Can you work these out from the drawing? Everything is in mm from the part's minimum corner. A direction names the side the tool comes from. Round coordinates to 2 decimals unless told otherwise and drop trailing zeros. Order: outer loops, then holes, each group sorted by start corner. A loop starts at its lowest first (then second) coordinate and runs counter-clockwise, first axis right, second up. Notation, with made-up numbers: (56, 23.5) - (92, 23.5) arc R22 cw to (92, 50.5) - close; hole circle Ø3 at (55.5, -4). An arc over 180 degrees is marked (long way). Answer as a JSON object with one key per item and string values.
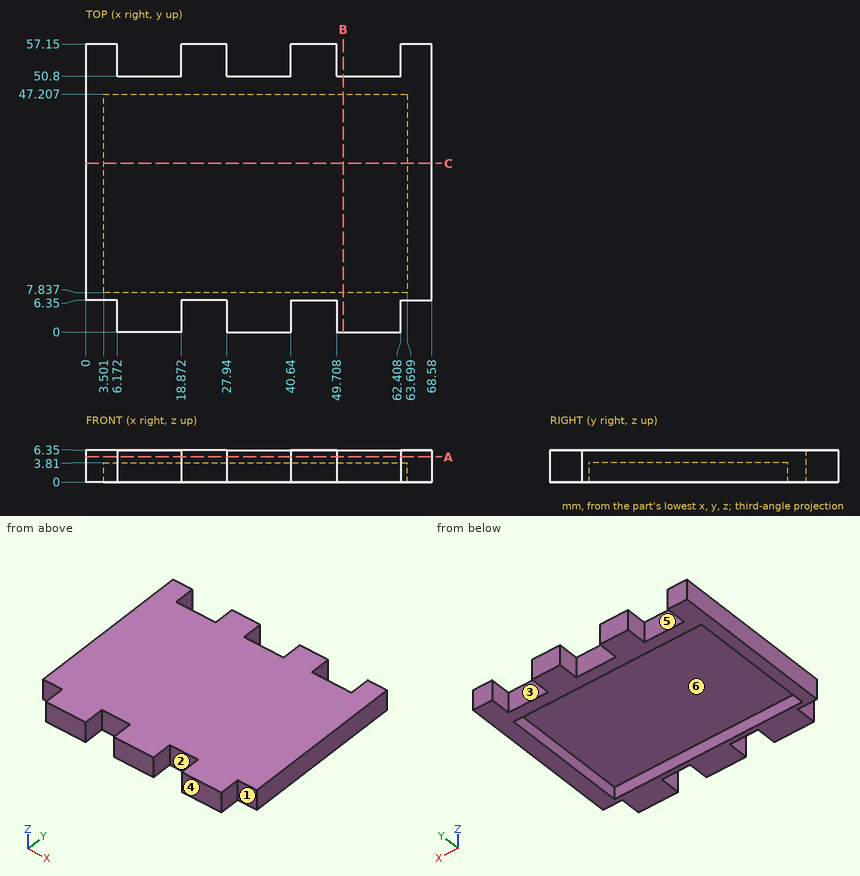
1. If I drill on L1, parallel to X at y = 3, z = 2; L2, parallel to X at y = 55.5, z = 5.5; L3, parallel to X at y = 29.5, z = 3, over which ranges is the centre line in solid material (lowest first)? Write a range as [from, to].
Responses:
{"L1": "[6.17, 18.87], [27.94, 40.64], [49.71, 62.41]", "L2": "[0, 6.17], [18.87, 27.94], [40.64, 49.71], [62.41, 68.58]", "L3": "[0, 3.5], [63.7, 68.58]"}
2. Imagine slicing it at A-A (z = 5). List the corners of the cut face in (x, y) for me, plus the area to 3 significant figures.
Responses:
{"outline": "(0, 6.35) - (6.17, 6.35) - (6.17, 0) - (18.87, 0) - (18.87, 6.35) - (27.94, 6.35) - (27.94, 0) - (40.64, 0) - (40.64, 6.35) - (49.71, 6.35) - (49.71, 0) - (62.41, 0) - (62.41, 6.35) - (68.58, 6.35) - (68.58, 57.15) - (62.41, 57.15) - (62.41, 50.8) - (49.71, 50.8) - (49.71, 57.15) - (40.64, 57.15) - (40.64, 50.8) - (27.94, 50.8) - (27.94, 57.15) - (18.87, 57.15) - (18.87, 50.8) - (6.17, 50.8) - (6.17, 57.15) - (0, 57.15) - close", "area": "3,480 mm2"}
3. Imagine slicing it at C-C (y = 33.5). List the corners of the cut face in (x, z) for me.
Responses:
{"outline": "(0, 0) - (3.5, 0) - (3.5, 3.81) - (63.7, 3.81) - (63.7, 0) - (68.58, 0) - (68.58, 6.35) - (0, 6.35) - close"}
4. For the marked faces 1, 2 and 3, which set-ups out of +Z, -Z, +X, -X, +Y, -Y let a thin tool reach every point of the face, with its end or its side?
Responses:
{"face 1": "+Z, -Z, +X, -Y", "face 2": "+Z, -Z, -Y", "face 3": "+Z, -Z, +Y"}
5. For P1, Ø3, axis at x = 9.5, z = 4, coming from the +Y side; P2, Ø1.9, axis at y = 2, z = 3, coming from the +X side; P3, Ø3, axis at x = 64, z = 4.5, coming from the -Y side, each with a flat end and sliding along its axis, tell me the tip position at first contact or that it passes through.
Responses:
{"P1": "y = 50.8", "P2": "x = 62.41", "P3": "y = 6.35"}
6. Imagine slicing it at B-B (x = 51). List the corners of the cut face in (y, z) for me.
Responses:
{"outline": "(0, 0) - (7.84, 0) - (7.84, 3.81) - (47.21, 3.81) - (47.21, 0) - (50.8, 0) - (50.8, 6.35) - (0, 6.35) - close"}
7. Thinking about a two-plate mould opening in Y: for the marked faces 4, 5 and 6, which applies, pulls with the +Y half, pulls with the -Y half, needs draft (parallel to the pull), parting line crosses it, or undercut?
Responses:
{"face 4": "pulls with the -Y half", "face 5": "pulls with the +Y half", "face 6": "undercut"}
